Geometry: final body of the model. Coordinates: model frame, mm. Face numbers are marked on the shaded views. Round coordinates to 2 decimals unless told otherwise and drop trailing zeros. Write each loop counter-clockwise with the first axis right and the second up, starting at its lowest first coordinate (ties: lowest second). Pieces come first, ordered by that corner, then holes.
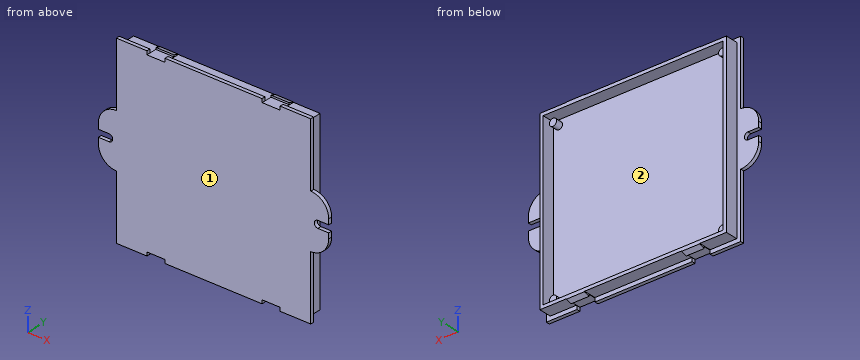
from build123d import *

# Parameters (mm, degrees)
SKETCH1_W            = 108
SKETCH1_H            = 102
BOSS_EXTRUDE1_DEPTH  = 2
SKETCH2_W            = 104
SKETCH2_H            = 98
BOSS_EXTRUDE2_DEPTH  = 7
SKETCH3_W            = 100
SKETCH3_H            = 94
CUT_EXTRUDE1_DEPTH   = 7
SKETCH4_W            = 10
SKETCH4_H            = 3
BOSS_EXTRUDE6_DEPTH  = 1
CUT_EXTRUDE2_DEPTH   = 10
SKETCH6_W            = 10
SKETCH6_H            = 3
BOSS_EXTRUDE7_DEPTH  = 1
CUT_EXTRUDE3_DEPTH   = 10
SKETCH9_W            = 10
SKETCH9_H            = 3
BOSS_EXTRUDE9_DEPTH  = 1
CUT_EXTRUDE4_DEPTH   = 10
SKETCH11_W           = 10
SKETCH11_H           = 3
BOSS_EXTRUDE10_DEPTH = 1
CUT_EXTRUDE5_DEPTH   = 10
SKETCH20_W           = 10
SKETCH20_H           = 2
CUT_EXTRUDE7_DEPTH   = 2
SKETCH21_W           = 10
SKETCH21_H           = 2
CUT_EXTRUDE8_DEPTH   = 2
SKETCH22_W           = 10
SKETCH22_H           = 2
CUT_EXTRUDE9_DEPTH   = 2
SKETCH23_W           = 10
SKETCH23_H           = 2
CUT_EXTRUDE11_DEPTH  = 2
SKETCH24_R           = 2
BOSS_EXTRUDE11_DEPTH = 4
BOSS_EXTRUDE12_DEPTH = 4
BOSS_EXTRUDE13_DEPTH = 4
BOSS_EXTRUDE14_DEPTH = 4
SKETCH28_W           = 30
SKETCH28_H           = 2
BOSS_EXTRUDE15_DEPTH = 10
SKETCH29_R           = 2
SKETCH29_W           = 6
SKETCH29_H           = 4
CUT_EXTRUDE12_DEPTH  = 2
FILLET1_R            = 10
SKETCH30_W           = 30
SKETCH30_H           = 1
BOSS_EXTRUDE16_DEPTH = 10
CUT_EXTRUDE13_DEPTH  = 2
FILLET2_R            = 10
SKETCH33_W           = 0.2
SKETCH33_H           = 98
CUT_EXTRUDE14_DEPTH  = 7
SKETCH34_W           = 14.8
SKETCH34_H           = 0.2
CUT_EXTRUDE15_DEPTH  = 7
SKETCH35_W           = 54
SKETCH35_H           = 0.2
CUT_EXTRUDE16_DEPTH  = 7
SKETCH36_W           = 15
SKETCH36_H           = 0.2
CUT_EXTRUDE17_DEPTH  = 7
SKETCH37_W           = 0.2
SKETCH37_H           = 97.8
CUT_EXTRUDE18_DEPTH  = 7
SKETCH39_W           = 14.8
SKETCH39_H           = 0.2
CUT_EXTRUDE19_DEPTH  = 7
SKETCH41_W           = 53.996290736
SKETCH41_H           = 0.2
CUT_EXTRUDE20_DEPTH  = 7
SKETCH42_W           = 14.8
SKETCH42_H           = 0.2
CUT_EXTRUDE21_DEPTH  = 7


with BuildPart() as part:
    # Sketch1 → Boss-Extrude1 (new body)
    with BuildSketch(Plane(origin=(0, 0, 0), x_dir=(1, 0, 0), z_dir=(0, 1, 0))):
        Rectangle(SKETCH1_W, SKETCH1_H)
    extrude(amount=BOSS_EXTRUDE1_DEPTH)

    # Sketch2 → Boss-Extrude2 (add)
    with BuildSketch(Plane(origin=(0, 2, 0), x_dir=(1, 0, 0), z_dir=(0, 1, 0))):
        Rectangle(SKETCH2_W, SKETCH2_H)
    extrude(amount=BOSS_EXTRUDE2_DEPTH)

    # Sketch3 → Cut-Extrude1 (cut)
    with BuildSketch(Plane(origin=(0, 9, 0), x_dir=(1, 0, 0), z_dir=(0, 1, 0))):
        Rectangle(SKETCH3_W, SKETCH3_H)
    extrude(amount=-CUT_EXTRUDE1_DEPTH, mode=Mode.SUBTRACT)

    # Sketch4 → Boss-Extrude6 (add)
    with BuildSketch(Plane.XY.offset(49)):
        with Locations((-32, 7.5)):
            Rectangle(SKETCH4_W, SKETCH4_H)
    extrude(amount=BOSS_EXTRUDE6_DEPTH)

    # Sketch5 → Cut-Extrude2 (cut)
    with BuildSketch(Plane(origin=(-27, 0, 0), x_dir=(0, 0, -1), z_dir=(1, 0, 0))):
        Polygon((-50, 6), (-49, 9), (-50, 9), align=None)
    extrude(amount=-CUT_EXTRUDE2_DEPTH, mode=Mode.SUBTRACT)

    # Sketch6 → Boss-Extrude7 (add)
    with BuildSketch(Plane.XY.offset(49)):
        with Locations((32, 7.5)):
            Rectangle(SKETCH6_W, SKETCH6_H)
    extrude(amount=BOSS_EXTRUDE7_DEPTH)

    # Sketch7 → Cut-Extrude3 (cut)
    with BuildSketch(Plane(origin=(37, 0, 0), x_dir=(0, 0, -1), z_dir=(1, 0, 0))):
        Polygon((-50, 6), (-49, 9), (-50, 9), align=None)
    extrude(amount=-CUT_EXTRUDE3_DEPTH, mode=Mode.SUBTRACT)

    # Sketch9 → Boss-Extrude9 (add)
    with BuildSketch(Plane(origin=(0, 0, -49), x_dir=(-1, 0, 0), z_dir=(0, 0, -1))):
        with Locations((-32, 7.5)):
            Rectangle(SKETCH9_W, SKETCH9_H)
    extrude(amount=BOSS_EXTRUDE9_DEPTH)

    # Sketch10 → Cut-Extrude4 (cut)
    with BuildSketch(Plane.ZY.offset(-27)):
        Polygon((-49, 9), (-50, 6), (-50, 9), align=None)
    extrude(amount=-CUT_EXTRUDE4_DEPTH, mode=Mode.SUBTRACT)

    # Sketch11 → Boss-Extrude10 (add)
    with BuildSketch(Plane(origin=(0, 0, -49), x_dir=(-1, 0, 0), z_dir=(0, 0, -1))):
        with Locations((32, 7.5)):
            Rectangle(SKETCH11_W, SKETCH11_H)
    extrude(amount=BOSS_EXTRUDE10_DEPTH)

    # Sketch12 → Cut-Extrude5 (cut)
    with BuildSketch(Plane.ZY.offset(37)):
        Polygon((-49, 9), (-50, 6), (-50, 9), align=None)
    extrude(amount=-CUT_EXTRUDE5_DEPTH, mode=Mode.SUBTRACT)

    # Sketch20 → Cut-Extrude7 (cut)
    with BuildSketch(Plane.XY.offset(51)):
        with Locations((32, 1)):
            Rectangle(SKETCH20_W, SKETCH20_H)
    extrude(amount=-CUT_EXTRUDE7_DEPTH, mode=Mode.SUBTRACT)

    # Sketch21 → Cut-Extrude8 (cut)
    with BuildSketch(Plane(origin=(0, 2, 0), x_dir=(1, 0, 0), z_dir=(0, 1, 0))):
        with Locations((-32, -50)):
            Rectangle(SKETCH21_W, SKETCH21_H)
    extrude(amount=-CUT_EXTRUDE8_DEPTH, mode=Mode.SUBTRACT)

    # Sketch22 → Cut-Extrude9 (cut)
    with BuildSketch(Plane(origin=(0, 2, 0), x_dir=(1, 0, 0), z_dir=(0, 1, 0))):
        with Locations((32, 50)):
            Rectangle(SKETCH22_W, SKETCH22_H)
    extrude(amount=-CUT_EXTRUDE9_DEPTH, mode=Mode.SUBTRACT)

    # Sketch23 → Cut-Extrude11 (cut)
    with BuildSketch(Plane(origin=(0, 2, 0), x_dir=(1, 0, 0), z_dir=(0, 1, 0))):
        with Locations((-32, 50)):
            Rectangle(SKETCH23_W, SKETCH23_H)
    extrude(amount=-CUT_EXTRUDE11_DEPTH, mode=Mode.SUBTRACT)

    # Sketch24 → Boss-Extrude11 (add)
    with BuildSketch(Plane(origin=(0, 2, 0), x_dir=(1, 0, 0), z_dir=(0, 1, 0))):
        with Locations(Location((47, 44, 0), (0, 0, 270))):
            Circle(SKETCH24_R)
    extrude(amount=BOSS_EXTRUDE11_DEPTH)

    # Sketch25 → Boss-Extrude12 (add)
    with BuildSketch(Plane(origin=(0, 2, 0), x_dir=(1, 0, 0), z_dir=(0, 1, 0))):
        with BuildLine():
            ThreePointArc((-45, 44), (-45.585786438, 45.414213562), (-47, 46))
            Line((-47, 46), (-47, 44))
            Line((-47, 44), (-49, 44))
            ThreePointArc((-49, 44), (-47, 42), (-45, 44))
        make_face()
        with BuildLine():
            Line((-47, 44), (-47, 46))
            ThreePointArc((-47, 46), (-48.414213562, 45.414213562), (-49, 44))
            Line((-49, 44), (-47, 44))
        make_face()
    extrude(amount=BOSS_EXTRUDE12_DEPTH)

    # Sketch26 → Boss-Extrude13 (add)
    with BuildSketch(Plane(origin=(0, 2, 0), x_dir=(1, 0, 0), z_dir=(0, 1, 0))):
        with BuildLine():
            ThreePointArc((-49, -44), (-48.414213562, -45.414213562), (-47, -46))
            Line((-47, -46), (-47, -44))
            Line((-47, -44), (-49, -44))
        make_face()
        with BuildLine():
            Line((-47, -44), (-47, -46))
            ThreePointArc((-47, -46), (-45.585786438, -45.414213562), (-45, -44))
            ThreePointArc((-45, -44), (-47, -42), (-49, -44))
            Line((-49, -44), (-47, -44))
        make_face()
    extrude(amount=BOSS_EXTRUDE13_DEPTH)

    # Sketch27 → Boss-Extrude14 (add)
    with BuildSketch(Plane(origin=(0, 2, 0), x_dir=(1, 0, 0), z_dir=(0, 1, 0))):
        with BuildLine():
            ThreePointArc((49, -44), (45.585786438, -42.585786438), (47, -46))
            Line((47, -46), (47, -44))
            Line((47, -44), (49, -44))
        make_face()
        with BuildLine():
            Line((47, -44), (47, -46))
            ThreePointArc((47, -46), (48.414213562, -45.414213562), (49, -44))
            Line((49, -44), (47, -44))
        make_face()
    extrude(amount=BOSS_EXTRUDE14_DEPTH)

    # Sketch28 → Boss-Extrude15 (add)
    with BuildSketch(Plane.ZY.offset(54)):
        with Locations((0, 1)):
            Rectangle(SKETCH28_W, SKETCH28_H)
    extrude(amount=BOSS_EXTRUDE15_DEPTH)

    # Sketch29 → Cut-Extrude12 (cut)
    with BuildSketch(Plane(origin=(0, 2, 0), x_dir=(1, 0, 0), z_dir=(0, 1, 0))):
        with Locations((-58, 0)):
            Circle(SKETCH29_R)
        with Locations((-61, 0)):
            Rectangle(SKETCH29_W, SKETCH29_H)
    extrude(amount=-CUT_EXTRUDE12_DEPTH, mode=Mode.SUBTRACT)

    # Fillet1
    fillet1_edges = [part.edges().sort_by_distance(p)[0] for p in [
        (-64, 1, 15),
        (-64, 1, -15),
    ]]
    fillet(fillet1_edges, radius=FILLET1_R - 0.0001)  # a hair under: the kernel refuses the full size

    # Sketch30 → Boss-Extrude16 (add)
    with BuildSketch(Plane(origin=(54, 0, 0), x_dir=(0, 0, -1), z_dir=(1, 0, 0))):
        with Locations((0, 1.5)):
            Rectangle(SKETCH30_W, SKETCH30_H)
        with Locations((0, 0.5)):
            Rectangle(SKETCH30_W, SKETCH30_H)
    extrude(amount=BOSS_EXTRUDE16_DEPTH)

    # Sketch32 → Cut-Extrude13 (cut)
    with BuildSketch(Plane(origin=(0, 2, 0), x_dir=(1, 0, 0), z_dir=(0, 1, 0))):
        with BuildLine():
            Line((58, -2), (64, -2))
            Line((64, -2), (64, 2))
            Line((64, 2), (58, 2))
            ThreePointArc((58, 2), (59.414213562, 1.414213562), (60, 0))
            ThreePointArc((60, 0), (59.414213562, -1.414213562), (58, -2))
        make_face()
        with BuildLine():
            ThreePointArc((58, 2), (56, 0), (58, -2))
            Line((58, -2), (58, 2))
        make_face()
        with BuildLine():
            Line((58, 2), (58, -2))
            ThreePointArc((58, -2), (59.414213562, -1.414213562), (60, 0))
            ThreePointArc((60, 0), (59.414213562, 1.414213562), (58, 2))
        make_face()
    extrude(amount=-CUT_EXTRUDE13_DEPTH, mode=Mode.SUBTRACT)

    # Fillet2
    fillet2_edges = [part.edges().sort_by_distance(p)[0] for p in [
        (64, 1, -15),
        (64, 1, 15),
    ]]
    fillet(fillet2_edges, radius=FILLET2_R - 0.0001)  # a hair under: the kernel refuses the full size

    # Sketch33 → Cut-Extrude14 (cut)
    with BuildSketch(Plane(origin=(0, 9, 0), x_dir=(1, 0, 0), z_dir=(0, 1, 0))):
        with Locations((51.9, 0)):
            Rectangle(SKETCH33_W, SKETCH33_H)
    extrude(amount=-CUT_EXTRUDE14_DEPTH, mode=Mode.SUBTRACT)

    # Sketch34 → Cut-Extrude15 (cut)
    with BuildSketch(Plane(origin=(0, 9, 0), x_dir=(1, 0, 0), z_dir=(0, 1, 0))):
        with Locations((44.4, 48.9)):
            Rectangle(SKETCH34_W, SKETCH34_H)
    extrude(amount=-CUT_EXTRUDE15_DEPTH, mode=Mode.SUBTRACT)

    # Sketch35 → Cut-Extrude16 (cut)
    with BuildSketch(Plane(origin=(0, 9, 0), x_dir=(1, 0, 0), z_dir=(0, 1, 0))):
        with Locations((0, 48.9)):
            Rectangle(SKETCH35_W, SKETCH35_H)
    extrude(amount=-CUT_EXTRUDE16_DEPTH, mode=Mode.SUBTRACT)

    # Sketch36 → Cut-Extrude17 (cut)
    with BuildSketch(Plane(origin=(0, 9, 0), x_dir=(1, 0, 0), z_dir=(0, 1, 0))):
        with Locations((-44.5, 48.9)):
            Rectangle(SKETCH36_W, SKETCH36_H)
    extrude(amount=-CUT_EXTRUDE17_DEPTH, mode=Mode.SUBTRACT)

    # Sketch37 → Cut-Extrude18 (cut)
    with BuildSketch(Plane(origin=(0, 9, 0), x_dir=(1, 0, 0), z_dir=(0, 1, 0))):
        with Locations((-51.9, -0.1)):
            Rectangle(SKETCH37_W, SKETCH37_H)
    extrude(amount=-CUT_EXTRUDE18_DEPTH, mode=Mode.SUBTRACT)

    # Sketch39 → Cut-Extrude19 (cut)
    with BuildSketch(Plane(origin=(0, 9, 0), x_dir=(1, 0, 0), z_dir=(0, 1, 0))):
        with Locations((-44.4, -48.9)):
            Rectangle(SKETCH39_W, SKETCH39_H)
    extrude(amount=-CUT_EXTRUDE19_DEPTH, mode=Mode.SUBTRACT)

    # Sketch41 → Cut-Extrude20 (cut)
    with BuildSketch(Plane(origin=(0, 9, 0), x_dir=(1, 0, 0), z_dir=(0, 1, 0))):
        with Locations((-0.001854632, -48.9)):
            Rectangle(SKETCH41_W, SKETCH41_H)
    extrude(amount=-CUT_EXTRUDE20_DEPTH, mode=Mode.SUBTRACT)

    # Sketch42 → Cut-Extrude21 (cut)
    with BuildSketch(Plane(origin=(0, 9, 0), x_dir=(1, 0, 0), z_dir=(0, 1, 0))):
        with Locations((44.4, -48.9)):
            Rectangle(SKETCH42_W, SKETCH42_H)
    extrude(amount=-CUT_EXTRUDE21_DEPTH, mode=Mode.SUBTRACT)


solid = part.part
1) Line query: probe 1 along Z at (x, y) = (-7.5, 8.5); probe 2 along X at (y, z) = (2.5, 6.5); probe 3 along Z at (x, y) = (-34, 2.25). Output: solid intervals per line, ascending.
2) Section B-B on z = -35. Output: boundary loops of the cut face in (x, y), plus the area to 3 significant figures.
3) Section C-C on x = -28.5. Output: boundary loops of the cut face in (y, z).
4) Draft query along Z for the marked faces 1 and 2. Return one class per face: pulls with the +Z half, pulls with the -Z half, needs draft (parallel to the pull), parting line crosses it, or undercut.
5) Section A-A on y = 4. Output: boundary loops of the cut face in (x, z).
6) First-contact query: P1, Ø2, axis at x = -6.5, y = 8, coming from the +Z side; P2, Ø2, axis at y = 7, z = -4, coming from the +X side; P3, Ø10, axis at x = -20.5, z = 8, coming from the +Y side; P4, Ø21.5, axis at x = -57, z = 13.5, coming from the +Y side. Flat tips, straight axial feed; report the tip coordinate or a pass-through.
Filled in:
1. probe 1: z = -48.8 to -47, 47 to 48.8
1. probe 2: x = -51.8 to -50, 50 to 51.8
1. probe 3: z = -49 to -47, 47 to 49
2. outline: (-54, 0) - (54, 0) - (54, 2) - (51.8, 2) - (51.8, 9) - (50, 9) - (50, 2) - (-50, 2) - (-50, 9) - (-51.8, 9) - (-51.8, 2) - (-54, 2) - close
2. area: 241 mm2
3. outline: (0, -49) - (6, -49) - (6, -50) - (9, -49) - (9, -47) - (2, -47) - (2, 47) - (9, 47) - (9, 49) - (6, 50) - (6, 49) - (0, 49) - close
4. face 1: needs draft
4. face 2: undercut
5. outline: (-51.8, -48.8) - (-37, -48.8) - (-37, -49) - (-27, -49) - (-27, -48.8) - (27, -48.8) - (27, -49) - (37, -49) - (37, -48.8) - (51.8, -48.8) - (51.8, 48.8) - (37, 48.8) - (37, 49) - (27, 49) - (27, 48.8) - (-27, 48.8) - (-27, 49) - (-37, 49) - (-37, 48.8) - (-51.8, 48.8) - close; circle Ø4 at (-47, -44); circle Ø4 at (-47, 44); circle Ø4 at (47, -44); circle Ø4 at (47, 44); hole (-50, -47) - (50, -47) - (50, 47) - (-50, 47) - close
6. P1: stops at z = 48.8
6. P2: stops at x = 51.8
6. P3: stops at y = 2
6. P4: stops at y = 9
